CAD build for the part. Positions are in the model's coordinates, mm. A direction names the side the tool comes from. Give positions to 0.01 mm unless a question says otherwise; leave off trailing zeros. Loops run counter-clockwise (first coordinate to the right, second up) from the corner with the lowest first, then second, coordinate; pieces in that order, holes last. Notation, with made-up numbers: M -18.75,-12.5 L 3.25,-12.5 A30 cw 3.25,21.5 Z; hole C 2,10 d6. An arc over 180 degrees is marked long. Answer as CSV lines item,"result".
```python
from build123d import *

# Parameters (mm, degrees)
SKETCH1_W           = 54
SKETCH1_H           = 33
BOSS_EXTRUDE1_DEPTH = 5
SKETCH4_R           = 1
BOSS_EXTRUDE2_DEPTH = 5
SKETCH6_R           = 1.5
CUT_EXTRUDE1_DEPTH  = 5


with BuildPart() as part:
    # Sketch1 → Boss-Extrude1 (new body)
    with BuildSketch(Plane(origin=(0, 0, 0), x_dir=(1, 0, 0), z_dir=(0, 1, 0))):
        with Locations((27, 16.5)):
            Rectangle(SKETCH1_W, SKETCH1_H)
    extrude(amount=BOSS_EXTRUDE1_DEPTH)

    # Sketch4 → Boss-Extrude2 (add)
    # profile 1 of 2: a face of its own
    with BuildSketch(Plane.XZ):
        with BuildLine():
            Line((62.748737342, -4.12233047), (54, -12.871067812))
            Line((54, -12.871067812), (54, 0))
            Line((54, 0), (52.728932188, 0))
            Line((52.728932188, 0), (55.67766953, 2.948737342))
            ThreePointArc((55.67766953, 2.948737342), (62.748737342, 2.948737342), (62.748737342, -4.12233047))
        make_face()
        with Locations(Location((59.213203436, -0.586796564, 0), (0, 0, 270))):
            Circle(SKETCH4_R, mode=Mode.SUBTRACT)
    # profile 2 of 2: a face of its own
    with BuildSketch(Plane.XZ):
        with BuildLine():
            Line((-8.748737342, -4.12233047), (0, -12.871067812))
            Line((0, -12.871067812), (0, 0))
            Line((0, 0), (1.271067812, 0))
            Line((1.271067812, 0), (-1.67766953, 2.948737342))
            ThreePointArc((-1.67766953, 2.948737342), (-8.748737342, 2.948737342), (-8.748737342, -4.12233047))
        make_face()
        with Locations(Location((-5.213203436, -0.586796564, 0), (0, 0, 270))):
            Circle(SKETCH4_R, mode=Mode.SUBTRACT)
    extrude(amount=-BOSS_EXTRUDE2_DEPTH)

    # Sketch6 → Cut-Extrude1 (cut)
    with BuildSketch(Plane.XZ):
        with Locations(Location((38, -21.8, 0), (0, 0, 270))):
            Circle(SKETCH6_R)
        with Locations(Location((16, -21.8, 0), (0, 0, 270))):
            Circle(SKETCH6_R)
    extrude(amount=-CUT_EXTRUDE1_DEPTH, mode=Mode.SUBTRACT)


solid = part.part
```
Q1. Cut at C-C (y = 1.1). Write the cut outline in (x, z), and give its area (3 significant figures).
Solution:
outline,"M -8.75,-4.12 L 0,-12.87 L 0,-33 L 54,-33 L 54,-12.87 L 62.75,-4.12 A5 ccw 55.68,2.95 L 52.73,0 L 1.27,0 L -1.68,2.95 A5 ccw Z; hole C -5.21,-0.59 d2; hole C 16,-21.8 d3; hole C 38,-21.8 d3; hole C 59.21,-0.59 d2"
area,"1,990 mm²"
Q2. Cut at A-A (z = -21.8). Write the cut outline in (x, y).
Solution:
outline,"M 0,0 L 14.5,0 L 14.5,5 L 0,5 Z; M 17.5,0 L 36.5,0 L 36.5,5 L 17.5,5 Z; M 39.5,0 L 54,0 L 54,5 L 39.5,5 Z"
Q3. Pin check, flat tips, straight feed: P1, Ø1, axis at y = 1.5, z = -17.5, coming from the -X side; P2, Ø1.5, axis at x = 39, y = 3, coming from the +Z side. Stop position of each tip, or through.
Solution:
P1,"stops at x = 0"
P2,"stops at z = 0"
Q4. Which spindle directions (+Z, -Z, +X, -X, +Y, -Y) get a long thin tool onto all of the face, cutting with end or side? Do faces 4 (the flat face through (-0.18, 2.46, 1.45)), 5 (the flat face through (0, 2, -23)), 6 (the cylindrical face through (58.237, 2.465, -0.37)). Say none if no direction does.
Solution:
face 4,"+Z, +Y, -Y"
face 5,"-Z, -X, +Y, -Y"
face 6,"+Y, -Y"
Q5. Wall check: line 1 (X direction, y = 2, z = -21.8); line 2 (X direction, y = 1.35, z = -22.5); line 3 (Z direction, x = 50.5, y = 4.2). Give the ranges that are in metal, low to high. Write a range as [from, to].
Solution:
line 1,"x = [0, 14.5], [17.5, 36.5], [39.5, 54]"
line 2,"x = [0, 14.67], [17.33, 36.67], [39.33, 54]"
line 3,"z = [-33, 0]"
Q6. Mould opens along Z. For faces 1 (the cylindrical face through (16.45, 2.46, -23.23)), 2 (the flat face through (54, 2, -23)), 3 (the flat face through (54.18, 2.46, 1.45)) say: released by +Z, released by -Z, zero draft, split by the parting line, or undercut.
Solution:
face 1,"undercut"
face 2,"zero draft"
face 3,"released by +Z"
Q7. Cut at D-D (z = -28). Write the cut outline in (x, y).
Solution:
outline,"M 0,0 L 54,0 L 54,5 L 0,5 Z"
Q8. Cut at B-B (x = 16). Write the cut outline in (y, z), and give its area (3 significant figures).
Solution:
outline,"M 0,-33 L 5,-33 L 5,-23.3 L 0,-23.3 Z; M 0,-20.3 L 5,-20.3 L 5,0 L 0,0 Z"
area,"150 mm²"
